Verification items for this drawing (mm, ordinates from the low corner). A direction names the side the tool comes from. Round coordinates to 2 decimals unless told otherwise and drop trailing zeros. Order: outer loops, then holes, each group sorted by start corner. A loop starts at its lowest first (then second) coordinate and runs counter-clockwise, first axis right, second up.
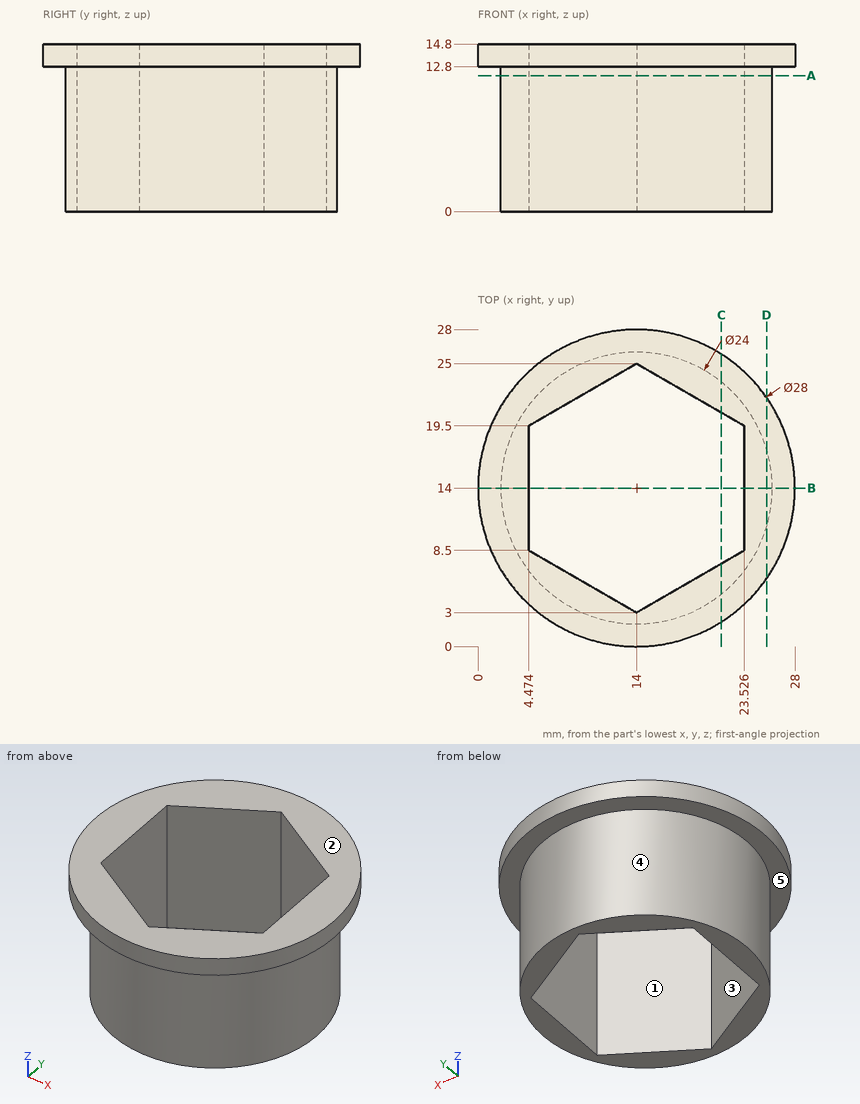
Item 1: Access from +Z, -Z, +X, -X, +Y, -Y to the whole of each face (thin tool, end or side, straight path). Record for the marked faces 1 and 2.
Answer:
face 1: +Z, -Z
face 2: +Z, +X, -X, +Y, -Y
Item 2: Sectioned sample at A-A (z = 12). Record the cut outline in (x, y).
Answer:
outline: circle Ø24 at (14, 14); hole (4.47, 8.5) - (14, 3) - (23.53, 8.5) - (23.53, 19.5) - (14, 25) - (4.47, 19.5) - close
Item 3: Release check for a two-part mould opening along X. For the marked faces 3, 4 and 5 record: released by +X, released by -X, zero draft, split by the parting line, or undercut.
Answer:
face 3: undercut
face 4: split by the parting line
face 5: zero draft
Item 4: Sectioned sample at C-C (x = 21.5). Record the cut outline in (y, z).
Answer:
outline: (2.18, 12.8) - (4.63, 12.8) - (4.63, 0) - (7.33, 0) - (7.33, 14.8) - (2.18, 14.8) - close; (20.67, 0) - (23.37, 0) - (23.37, 12.8) - (25.82, 12.8) - (25.82, 14.8) - (20.67, 14.8) - close
Item 5: Scan lines: line 1 along X through (y, z) = (18.5, 11.5) (1 decimal); line 2 along X through (y, z) = (6.5, 13.5); line 3 along Z through (x, y) = (2.5, 9.5). Record each from-to range of solid material in increasing order.
Answer:
line 1: x = 2.9 to 4.5, 23.5 to 25.1
line 2: x = 2.18 to 7.94, 20.06 to 25.82
line 3: z = 12.8 to 14.8
Item 6: Sectioned sample at D-D (x = 25.5). Record the cut outline in (y, z).
Answer:
outline: (6.02, 12.8) - (10.57, 12.8) - (10.57, 0) - (17.43, 0) - (17.43, 12.8) - (21.98, 12.8) - (21.98, 14.8) - (6.02, 14.8) - close
Item 7: Sectioned sample at B-B (y = 14). Record the cut outline in (x, z).
Answer:
outline: (0, 12.8) - (2, 12.8) - (2, 0) - (4.47, 0) - (4.47, 14.8) - (0, 14.8) - close; (23.53, 0) - (26, 0) - (26, 12.8) - (28, 12.8) - (28, 14.8) - (23.53, 14.8) - close
Item 8: Go/stop test with flat-tipped pins: P1, Ø1, axis at y = 8.5, z = 3, coming from the +X side; P2, Ø4, axis at x = 11, z = 4, coming from the -Y side; P3, Ø3.5, axis at y = 12.5, z = 7.5, coming from the -X side. Record where each tip stops, or that it passes through.
Answer:
P1: stops at x = 24.91
P2: stops at y = 2.04
P3: stops at x = 2
